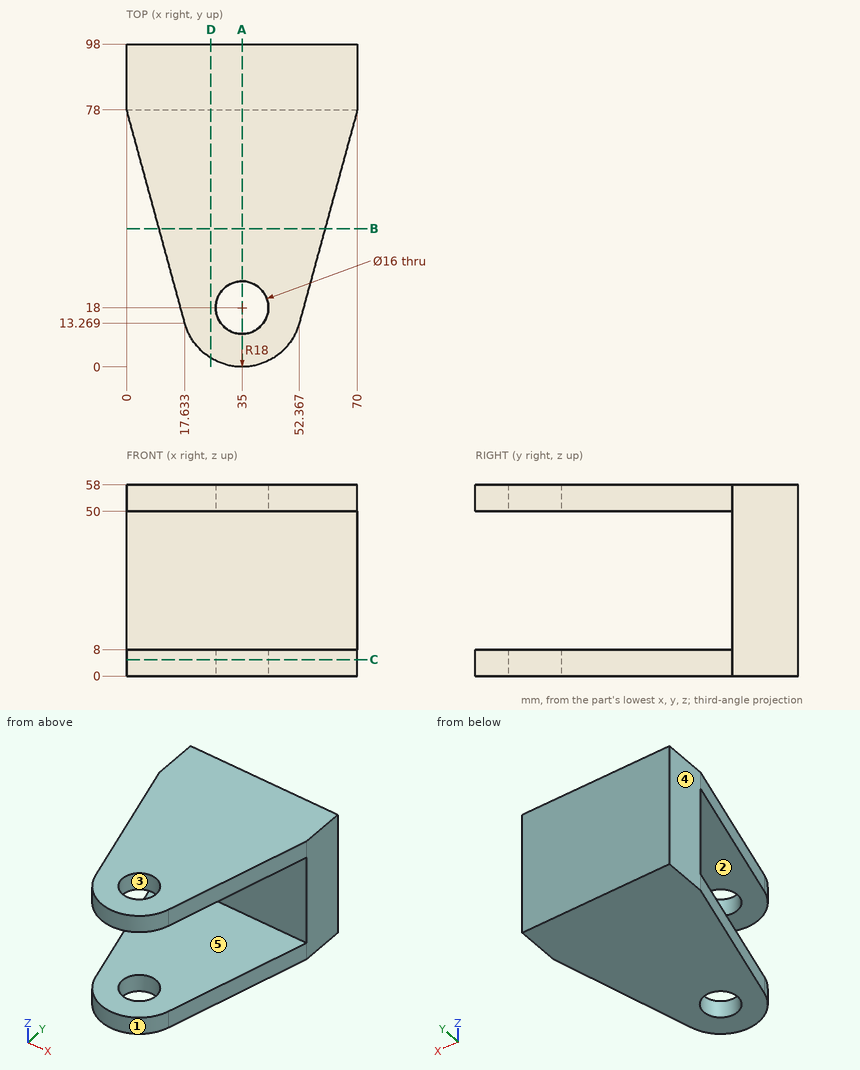
For this review, use the dimensioned drawing (mm, ordinates from the lowest corner) and the shaded views. A direction names the side the tool comes from. Give positions to 0.01 mm unless a question says otherwise; leave off trailing zeros. Order: outer loops, then holes, each group sorted by start corner. A loop starts at its lowest first (then second) coordinate and runs counter-clockwise, first axis right, second up. Notation, with made-up numbers: (57, -22) - (108, -22) arc R15 cw to (108, -16) - close; hole circle Ø9 at (88.25, -10). An arc over 180 degrees is marked (long way). Use CSV: the item, a comma, the result in double quotes. Start each with the question number.
Q1. Take a section at A-A (x = 35). State the section outline as (y, z) points.
Q2. For line 1 (Y direction, x = 35, z = 52.5); line 2 (Z direction, x = 46.5, y = 59); line 3 (Y direction, x = 48, z = 34), list the stretches that pass through material, from the lowest coordinate up.
Q3. Draft analysis for pull direction X (two halves, no side actions). For the marked faces 1, 2 and 3, state which applies: pulls with the +X half, pulls with the -X half, needs draft (parallel to the pull), parting line crosses it, or undercut.
Q4. Take a section at D-D (x = 25.5). State the section outline as (y, z) points.
Q5. Machinability: for the marked faces 4 and 5, which of the approach directions +Z, -Z, +X, -X, +Y, -Y give a long, thin tool a straight path to every point of the face, cutting with its end or side? Answer none if there is none.
Q6. Take a section at C-C (z = 5). State the section outline as (x, y) points.
Q7. For P1, Ø1.5, axis at y = 12.5, z = 8, coming from the +X side, flat-tipped, find the tip position at first contact; note if it passes through.
Q8. Take a section at B-B (y = 42). State the section outline as (x, z) points, and give its area (3 significant figures).
Calculated:
1,outline,"(0, 0) - (10, 0) - (10, 8) - (0, 8) - close; (0, 50) - (10, 50) - (10, 58) - (0, 58) - close; (26, 0) - (98, 0) - (98, 58) - (26, 58) - (26, 50) - (78, 50) - (78, 8) - (26, 8) - close"
2,line 1,"y = 0 to 10, 26 to 98"
2,line 2,"z = 0 to 8, 50 to 58"
2,line 3,"y = 78 to 98"
3,face 1,"parting line crosses it"
3,face 2,"needs draft"
3,face 3,"undercut"
4,outline,"(2.71, 0) - (98, 0) - (98, 58) - (2.71, 58) - (2.71, 50) - (78, 50) - (78, 8) - (2.71, 8) - close"
5,face 4,"+Z, -Z, -X, +Y, -Y"
5,face 5,"+X, -X, -Y"
6,outline,"(0, 78) - (17.63, 13.27) arc R18 ccw to (52.37, 13.27) - (70, 78) - (70, 98) - (0, 98) - close; hole circle Ø16 at (35, 18)"
7,P1,"stops at x = 52.36"
8,outline,"(9.81, 0) - (60.19, 0) - (60.19, 8) - (9.81, 8) - close; (9.81, 50) - (60.19, 50) - (60.19, 58) - (9.81, 58) - close"
8,area,"806 mm²"
